Part print with two shaded views. Sizes in mm from the minimum x, y, z corner. Coordinates: 2 decimals unless noted, no trailing zeros. Loops run counter-clockwise (first coordinate to the right, second up) from the corner with the lowest first, then second, coordinate; pieces in that order, holes last.
(1) Flat gauge pin, fed straight in: P1, Ø3, axis at x = 173.2, y = 7.894, coming from the -Z side. Where does the tip first touch, or does it go through?
(2) Slice it at A-A (y = 95). Give the cut face in (x, z).
(3) Wall check: L1, parallel to X at y = 79.5, z = 1.6; L2, parallel to Y at x = 116.5, z = 0.6 (1 decimal). Give the ranges that are in metal, low to high.
(4) Slice it at C-C (z = 1.55). Give the number of separate pieces and of enclosed holes in the cut face, and give its area (3 significant figures).
(5) Slice it at B-B (x = 102.5). Give the cut face in (y, z) (1 decimal), and give its area (3 significant figures).
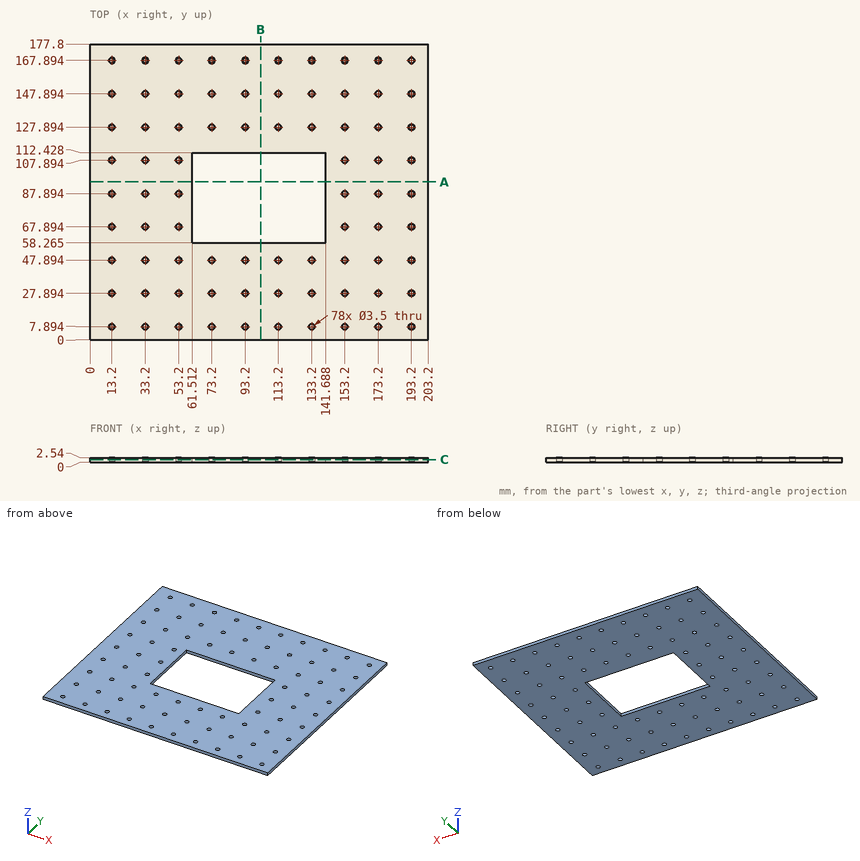
Response values:
1. P1: passes through
2. outline: (0, 0) - (61.51, 0) - (61.51, 2.54) - (0, 2.54) - close; (141.69, 0) - (203.2, 0) - (203.2, 2.54) - (141.69, 2.54) - close
3. L1: x = 0 to 61.51, 141.69 to 203.2
3. L2: y = 0 to 58.3, 112.4 to 177.8
4. separate pieces: 1
4. enclosed holes: 79
4. area: 31,000 mm2
5. outline: (0, 0) - (58.3, 0) - (58.3, 2.5) - (0, 2.5) - close; (112.4, 0) - (177.8, 0) - (177.8, 2.5) - (112.4, 2.5) - close
5. area: 314 mm2
